Geometry: final body of the model. Coordinates: model frame, mm. Round coordinates to 2 decimals unless told otherwise and drop trailing zeros. Loops run counter-clockwise (first coordinate to the right, second up) from the corner with the lowest first, then second, coordinate; pieces in that order, holes last. Notation, with made-up numbers: (8, 22) - (59, 22) arc R12 ccw to (59, 35) - close; hole circle Ø11 at (-26.75, 23). An arc over 180 degrees is marked (long way). Use CSV: the item, a comma, the result in double quotes.
from build123d import *

# Parameters (mm, degrees)
IZIM1_R                     = 47.5
IZIM1_R_2                   = 9.5
Y_KSEKLIK_EKSTR_ZYON1_DEPTH = 63


with BuildPart() as part:
    # Çizim1 → Yükseklik-Ekstrüzyon1 (new body)
    with BuildSketch(Plane.XY):
        Circle(IZIM1_R)
        Circle(IZIM1_R_2, mode=Mode.SUBTRACT)
        with BuildLine():
            Line((30.56284509, 4.75), (15.896540504, 4.75))
            ThreePointArc((15.896540504, 4.75), (13.947181635, 5.288098714), (12.549900398, 6.75))
            ThreePointArc((12.549900398, 6.75), (10.076271632, 10.076271632), (6.75, 12.549900398))
            ThreePointArc((6.75, 12.549900398), (5.288098714, 13.947181635), (4.75, 15.896540504))
            Line((4.75, 15.896540504), (4.75, 30.56284509))
            ThreePointArc((4.75, 30.56284509), (7.134994011, 35.199733626), (12.294117647, 35.956288341))
            ThreePointArc((12.294117647, 35.956288341), (26.870057685, 26.870057685), (35.956288341, 12.294117647))
            ThreePointArc((35.956288341, 12.294117647), (35.199733626, 7.134994011), (30.56284509, 4.75))
        make_face(mode=Mode.SUBTRACT)
        with BuildLine():
            Line((-30.56284509, 4.75), (-15.896540504, 4.75))
            ThreePointArc((-15.896540504, 4.75), (-13.947181635, 5.288098714), (-12.549900398, 6.75))
            ThreePointArc((-12.549900398, 6.75), (-10.076271632, 10.076271632), (-6.75, 12.549900398))
            ThreePointArc((-6.75, 12.549900398), (-5.288098714, 13.947181635), (-4.75, 15.896540504))
            Line((-4.75, 15.896540504), (-4.75, 30.56284509))
            ThreePointArc((-4.75, 30.56284509), (-7.134994011, 35.199733626), (-12.294117647, 35.956288341))
            ThreePointArc((-12.294117647, 35.956288341), (-26.870057685, 26.870057685), (-35.956288341, 12.294117647))
            ThreePointArc((-35.956288341, 12.294117647), (-35.199733626, 7.134994011), (-30.56284509, 4.75))
        make_face(mode=Mode.SUBTRACT)
        with BuildLine():
            Line((4.75, -30.56284509), (4.75, -15.896540504))
            ThreePointArc((4.75, -15.896540504), (5.288098714, -13.947181635), (6.75, -12.549900398))
            ThreePointArc((6.75, -12.549900398), (10.076271632, -10.076271632), (12.549900398, -6.75))
            ThreePointArc((12.549900398, -6.75), (13.947181635, -5.288098714), (15.896540504, -4.75))
            Line((15.896540504, -4.75), (30.56284509, -4.75))
            ThreePointArc((30.56284509, -4.75), (35.199733626, -7.134994011), (35.956288341, -12.294117647))
            ThreePointArc((35.956288341, -12.294117647), (26.870057685, -26.870057685), (12.294117647, -35.956288341))
            ThreePointArc((12.294117647, -35.956288341), (7.134994011, -35.199733626), (4.75, -30.56284509))
        make_face(mode=Mode.SUBTRACT)
        with BuildLine():
            Line((-30.56284509, -4.75), (-15.896540504, -4.75))
            ThreePointArc((-15.896540504, -4.75), (-13.947181635, -5.288098714), (-12.549900398, -6.75))
            ThreePointArc((-12.549900398, -6.75), (-10.076271632, -10.076271632), (-6.75, -12.549900398))
            ThreePointArc((-6.75, -12.549900398), (-5.288098714, -13.947181635), (-4.75, -15.896540504))
            Line((-4.75, -15.896540504), (-4.75, -30.56284509))
            ThreePointArc((-4.75, -30.56284509), (-7.134994011, -35.199733626), (-12.294117647, -35.956288341))
            ThreePointArc((-12.294117647, -35.956288341), (-26.870057685, -26.870057685), (-35.956288341, -12.294117647))
            ThreePointArc((-35.956288341, -12.294117647), (-35.199733626, -7.134994011), (-30.56284509, -4.75))
        make_face(mode=Mode.SUBTRACT)
    extrude(amount=Y_KSEKLIK_EKSTR_ZYON1_DEPTH)


solid = part.part
Item 1: Pin query (flat end, axial travel): P1, Ø11.5, axis at y = -21.5, z = 46.5, coming from the +X side; P2, Ø4.5, axis at y = 23.5, z = 17.5, coming from the -X side; P3, Ø3, axis at y = 21, z = 49.5, coming from the +X side; P4, Ø11.5, axis at x = 0, y = 0, coming from the +Z side. Return the tip coordinate at first contact, or that it passes through.
Final values:
P1,"stops at x = 44.81"
P2,"stops at x = -42.48"
P3,"stops at x = 43.31"
P4,"passes through"
Item 2: Material intervals for line 1 (X direction, y = 11, z = 5); line 2 (Y direction, x = 7.5, z = 38.5); line 3 (X direction, y = -18, z = 44.5), sorted ascending.
Final values:
line 1,"x = -46.21 to -36.24, -9.06 to 9.06, 36.24 to 46.21"
line 2,"y = -46.9 to -35.44, -12.12 to -5.83, 5.83 to 12.12, 35.44 to 46.9"
line 3,"x = -43.96 to -33.47, -4.75 to 4.75, 33.47 to 43.96"
Item 3: Mould query, pull axis X, two halves, no side actions, for faces 1 (the flat face through (10, 1, 63)), 2 (the cylindrical face through (-13.972, 5.273, 31.059)), 3 (the cylindrical face through (-7.074, 35.155, 31.059)). Classes: released by +X, released by -X, zero draft, split by the parting line, or undercut.
Final values:
face 1,"zero draft"
face 2,"undercut"
face 3,"undercut"
Item 4: Section D-D on y = 11. Return the cut outline in (x, z), plus the area to 3 significant figures.
Final values:
outline,"(-46.21, 0) - (-36.24, 0) - (-36.24, 63) - (-46.21, 63) - close; (-9.06, 0) - (9.06, 0) - (9.06, 63) - (-9.06, 63) - close; (36.24, 0) - (46.21, 0) - (46.21, 63) - (36.24, 63) - close"
area,"2,400 mm²"
Item 5: Section A-A on y = 0. Return the cut outline in (x, z), plus the area to 3 significant figures.
Final values:
outline,"(-47.5, 0) - (-9.5, 0) - (-9.5, 63) - (-47.5, 63) - close; (9.5, 0) - (47.5, 0) - (47.5, 63) - (9.5, 63) - close"
area,"4,790 mm²"
Item 6: Section B-B on z = 37. Give the number of separate pieces and of enclosed holes in the cut face, plus the area to 3 significant figures.
Final values:
separate pieces,"1"
enclosed holes,"5"
area,"3,920 mm²"
